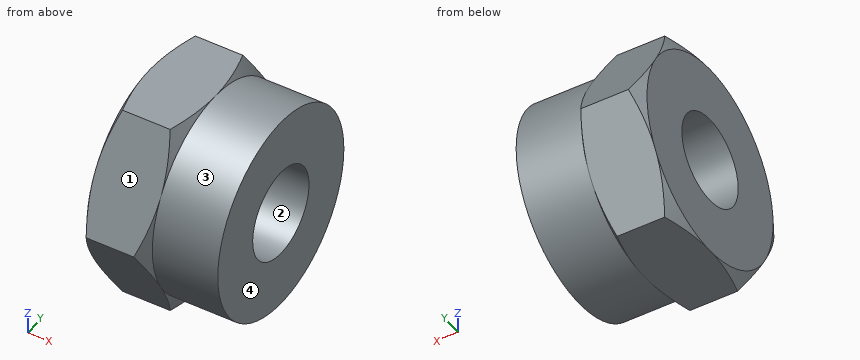
Autodesk Inventor part; units mm, degrees
ref_plane "Work Plane1" through (9.1402, 0, 0) normal (0, 0, -1) x (-1, 0, 0)
ref_plane "YZ Plane" through (0, 0, 0) normal (1, 0, 0) x (0, 1, 0)
ref_plane "XZ Plane" through (0, 0, 0) normal (0, 1, 0) x (-1, 0, 0)
sketch "Szkic1" plane through (0, 0, 0) normal (1, 0, 0) x (0, 1, 0)
  line L0 (3.1754, 0) -> (1.5877, -2.75)
  line L1 (1.5877, -2.75) -> (-1.5877, -2.75)
  line L2 (-1.5877, -2.75) -> (-3.1754, 0)
  line L3 (-3.1754, 0) -> (-1.5877, 2.75)
  line L4 (-1.5877, 2.75) -> (1.5877, 2.75)
  line L5 (1.5877, 2.75) -> (3.1754, 0)
  point P0 (0, 0)
  point P1 (0, 0)
  dimension "d0" = 5.5
extrude "Głowica" add sketch "Szkic1" along normal blind 1.8
sketch "Szkic2" plane through (0, 0, 0) normal (0, 0, 1) x (1, 0, 0)
  line L0 (3.6, 0) -> (3.6, 2.75)
  line L1 (3.6, 2.75) -> (1.8, 2.75)
  line L2 (1.8, 0) -> (3.6, 0)
  line L3 (0, -0.55) -> (0, 3.3)
  line L4 (1.8, 0) -> (1.8, 2.75)
  line L5 (1.44, 0) -> (3.96, 0)
  dimension "d3" = 5.5
  dimension "d4" = 5.5
  dimension "d5" = 3.6
  dimension "d6" = 1.8
revolve "Bryła" add sketch "Szkic2" angle 360 about axis through (1.8, 0, 0) along (1, 0, 0)
sketch "Szkic3" plane through (0, 0, 0) normal (-1, 0, 0) x (0, 0, 1)
  point P0 (0, 0)
hole "Gwint" at (0, 0, 0) direction (1, 0, 0) diameter 2.459 end through all
sketch "Szkic4" plane through (0, 0, 0) normal (0, 0, 1) x (1, 0, 0)
  line L0 (1.8, 2.75) -> (1.8, 3.1754)
  line L1 (1.8, 3.1754) -> (1.5544, 3.1754)
  line L2 (1.5544, 3.1754) -> (1.8, 2.75)
  line L3 (0.2456, 3.1754) -> (0, 3.1754)
  line L4 (0, 3.1754) -> (0, 2.75)
  line L5 (0, 2.75) -> (0.2456, 3.1754)
  line L6 (1.8, 3.1754) -> (1.8, 2.3816)
  line L7 (0, 3.1754) -> (1.8, 3.1754)
  line L8 (0, 3.1754) -> (0, 1.5877)
  line L9 (-0.36, 0) -> (2.16, 0)
  dimension "d7" = 5.5
  dimension "d8" = 5.5
  dimension "d9" = 30
  dimension "d10" = 30
revolve "Faza1" cut sketch "Szkic4" angle 360 about axis through (-10, 0, 0) along (1, 0, 0)
ref_plane "Work Plane1" through (9.1402, 0, 0) normal (0, 0, -1) x (-1, 0, 0)
equation "\"d0\" = SW"
equation "\"d1\" = KOH1"
equation "\"d3\" = SW"
equation "\"d4\" = SW0"
equation "\"d5\" = KOH"
equation "\"d6\" = KOH1"
equation "\"d7\" = SW"
equation "\"d8\" = SW"
equation "\"d9\" = ANG1"
equation "\"d10\" = ANG2"
equation "\"SW\" = 5.5"
equation "\"KOH\" = 3.6"
equation "\"SW0\" = SW"
equation "\"ANG1\" = 30deg"
equation "\"ANG2\" = 30deg"
equation "\"KOH1\" = 1.8"
equation "\"GUL\" = 0.541266 * PTC"
equation "\"WFT\" = 0.4"
equation "\"PDM\" = 4.8"
equation "\"SDH\" = SW"
equation "\"TOA\" = 30deg"
equation "\"PTC\" = 0.5"
equation "\"NND\" = 3"
equation "\"THREADDIA\" = 3"
equation "\"GAL\" = 0.541266 * PTC"
equation "\"E0\" = 1.155 * SW"
properties part number "AS 1285 - M3" material "Stal, miękka"
Model file for the job. Use its own axes, mm. Face numbers are marked on the shaded views. Round coordinates to 2 decimals unless told otherwise and drop trailing zeros. Loops run counter-clockwise (first coordinate to the right, second up) from the corner with the lowest first, then second, coordinate; pieces in that order, holes last. Notation, with made-up numbers: M 57.25,34.5 L 111.25,34.5 A13 ccw 111.25,39.5 Z; hole C 68,62.25 d3. An arc over 180 degrees is marked long. Put each result on its own line as item: value. Start each with the question number.
Item 1: Drill centre line: line 1 along Z through (x, y) = (1.55, 0). Where is it in solid material? Low to high.
Item 2: Mould opens along Y. For the marked faces 1, 2, 3 and 4 say: released by +Y, released by -Y, zero draft, split by the parting line, or undercut.
Item 3: Cut at B-B (x = 2.6). List the corners of the cut face in (y, z).
Item 4: Cut at A-A (x = 0.8). List the corners of the cut face in (y, z), then the cut area to 3 significant figures.
Item 5: Drop flat-ended pins along their axis: P1, Ø1, axis at x = 1.5, z = 1.5, coming from the +Y side; P2, Ø2, axis at y = 0, z = 0, coming from the -X side; P3, Ø1, axis at x = 0.5, z = -1, coming from the +Y side; P4, Ø1.5, axis at x = 2, y = 2, coming from the -Z side. Give the stop position or say it passes through.
Answer block:
1. line 1: -2.75 to -1.23, 1.23 to 2.75
2. face 1: released by -Y
2. face 2: undercut
2. face 3: split by the parting line
2. face 4: zero draft
3. outline: C 0,0 d5.5; hole C 0,0 d2.46
4. outline: M -3.18,0 L -1.59,-2.75 L 1.59,-2.75 L 3.18,0 L 1.59,2.75 L -1.59,2.75 Z; hole C 0,0 d2.46
4. area: 21.4 mm2
5. P1: y = 2.6
5. P2: through
5. P3: y = 2.89
5. P4: z = -2.75
